Geometry: see drawing. Coordinates: mm, zero at the bounding-box minimum. A direction names the side the tool comes from. Round coordinates to 2 decimals unless told otherwise and drop trailing zeros. Order: outer loops, then holes, each group sorted by start corner. A loop starts at its lowest first (then second) coordinate and runs counter-clockwise, first axis right, second up. Notation, with made-up numbers: (81, 71.25) - (85, 71.25) arc R17 ccw to (85, 86.25) - close; hole circle Ø9 at (85, 86.5). An arc over 180 degrees is marked (long way). Put each result on its own line as item: value. Start each with the question number.
1) Contact query for flat-ended pins moving along their axis: P1, Ø6, axis at x = 25.5, z = 6.5, coming from the -Y side; P2, Ø5, axis at x = 14, y = 11, coming from the +Z side; P3, Ø4, axis at x = 26, z = 11.5, coming from the -Y side. Output: stop coordinate, or through.
2) Line query: probe 1 along X at (y, z) = (6.25, 1); probe 2 along Y at (x, z) = (13, 6.5); probe 3 along Z at (x, y) = (38.5, 10). Output: solid intervals per line, ascending. Write a range as [from, to].
3) Access query for the marked faces 1 and 2. Directions: +Z, -Z, +X, -X, +Y, -Y. A direction counts if a zero-diameter tool reaches every point of the face in a straight line with its end or side. Return the directions, or none.
4) Section A-A on x = 25.5. Output: boundary loops of the cut face in (y, z).
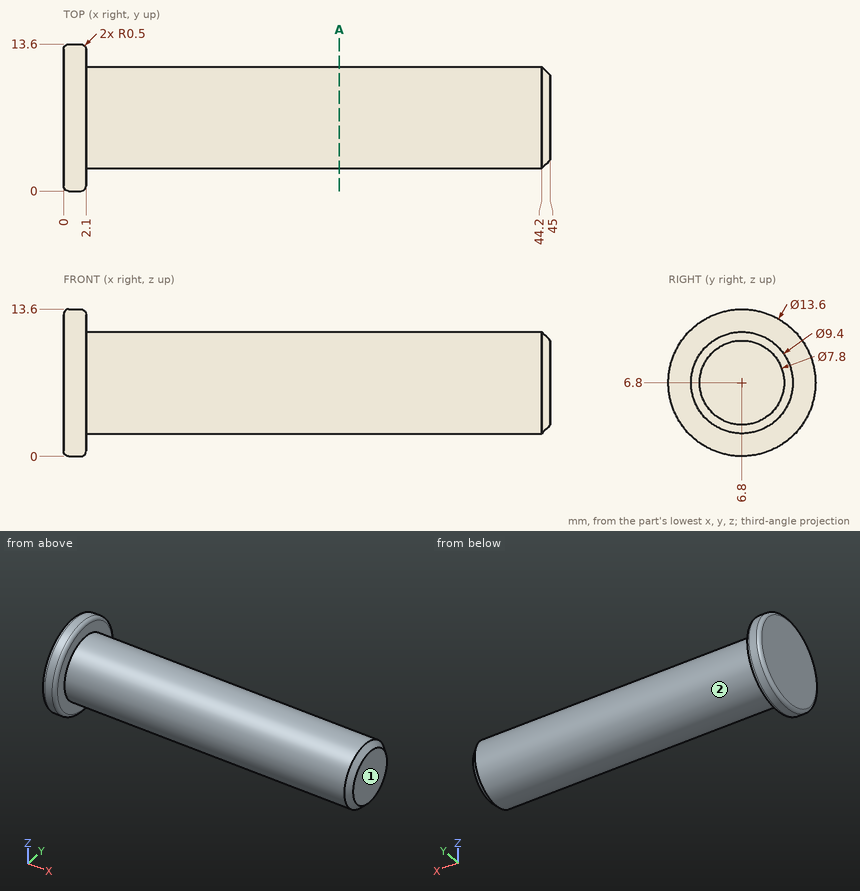
Answer sheet:
1. P1: y = 2.1
1. P2: z = 11.18
1. P3: y = 2.95
2. probe 1: [0, 2.1]
2. probe 2: [2.11, 11.49]
2. probe 3: [3.36, 10.24]
3. face 1: +Z, -Z, +X, +Y, -Y
3. face 2: +X
4. outline: circle Ø9.4 at (6.8, 6.8)
